Design review of the part built by this model. Coordinates are the model's own, in mm. A direction names the side the tool comes from. Round coordinates to 2 decimals unless told otherwise and drop trailing zeros. Loops run counter-clockwise (first coordinate to the right, second up) from the corner with the lowest first, then second, coordinate; pieces in that order, holes last. Notation, with made-up numbers: (86, -8) -> (128, -8) arc R21 ccw to (128, 29) -> close; hole circle Ø8 at (33, 54). An arc over 180 degrees is marked (long way). Answer as CSV lines item,"result". Start each with the question number.
```python
from build123d import *

# Parameters (mm, degrees)
PAD023_DEPTH     = 30
POCKET022_DEPTH  = 203.460811
POCKET023_DEPTH  = 25.001
SKETCH049_W      = 110.6
SKETCH049_H      = 62.6
POCKET024_DEPTH  = 33.001
SKETCH051_W      = 120.3
SKETCH051_H      = 69.7
POCKET025_DEPTH  = 2
CHAMFER001_SIZE2 = 2
CHAMFER001_SIZE  = 4
SKETCH054_R      = 1.25
POCKET029_DEPTH  = 7.001
SKETCH052_R      = 3
POCKET030_DEPTH  = 3


with BuildPart() as part:
    # Sketch045 → Pad023 (new body)
    with BuildSketch(Plane.XZ.offset(7)):
        with BuildLine():
            ThreePointArc((-100.852547, 31.281341), (-87.977329, 12.342987), (-66.272551, 5.039896))
            Line((-66.272551, 5.039896), (66.272551, 5.039896))
            ThreePointArc((66.272551, 5.039896), (87.977329, 12.342987), (100.852547, 31.281341))
            ThreePointArc((100.852547, 31.281341), (100.091262, 61.855424), (91.843705, 91.305923))
            ThreePointArc((34.688969, 97.850786), (63.036347, 92.569904), (91.843705, 91.305923))
            ThreePointArc((34.688969, 97.850786), (0, 104.060193), (-34.688969, 97.850786))
            ThreePointArc((-91.843705, 91.305923), (-63.036347, 92.569904), (-34.688969, 97.850786))
            ThreePointArc((-91.843705, 91.305923), (-100.091262, 61.855424), (-100.852547, 31.281341))
        make_face()
    extrude(amount=PAD023_DEPTH)

    # Sketch048 → Pocket022 (cut, through all)
    with BuildSketch(Plane.YZ.offset(102)):
        with BuildLine():
            ThreePointArc((-12, 23.34), (-23.12479, 56.152072), (-39.155961, 86.866801))
            Line((-39.155961, 23.34), (-39.155961, 86.866801))
            Line((-39.155961, 23.34), (-12, 23.34))
        make_face()
    extrude(amount=-POCKET022_DEPTH, mode=Mode.SUBTRACT)

    # Sketch050 → Pocket023 (cut, through all)
    with BuildSketch(Plane.XZ.offset(12)):
        with BuildLine():
            ThreePointArc((-86.154363, 83.544791), (-58.846051, 86.250597), (-32.141142, 92.568282))
            ThreePointArc((32.141142, 92.568282), (0, 97.874317), (-32.141142, 92.568282))
            ThreePointArc((32.141142, 92.568282), (58.846051, 86.250597), (86.154363, 83.544791))
            ThreePointArc((93.603594, -14.330003), (97.449111, 35.183555), (86.154363, 83.544791))
            Line((-93.603594, -14.330003), (93.603594, -14.330003))
            ThreePointArc((-86.154363, 83.544791), (-98.508002, 35.264147), (-93.603594, -14.330003))
        make_face()
    extrude(amount=POCKET023_DEPTH, mode=Mode.SUBTRACT)

    # Sketch049 → Pocket024 (cut, through all)
    with BuildSketch(Plane.XZ.offset(4)):
        with Locations((0, 41.080998)):
            Rectangle(SKETCH049_W, SKETCH049_H)
    extrude(amount=POCKET024_DEPTH, mode=Mode.SUBTRACT)

    # Sketch051 → Pocket025 (cut)
    with BuildSketch(Plane(origin=(0, -7, 41), x_dir=(1, 0, 0), z_dir=(0, -1, 0))):
        with Locations((-3.04, -0.08)):
            Rectangle(SKETCH051_W, SKETCH051_H)
    extrude(amount=POCKET025_DEPTH, mode=Mode.SUBTRACT)

    # Chamfer001
    chamfer001_edges = [part.edges().sort_by_distance(p)[0] for p in [
        (55.3, -12, 41.080998),
        (0, -12, 72.380998),
        (-55.3, -12, 41.080998),
        (0, -12, 9.780998),
    ]]
    chamfer001_side = part.faces().sort_by_distance((-83.299387, -12, 11.829323))[0]
    chamfer(chamfer001_edges, length=CHAMFER001_SIZE, length2=CHAMFER001_SIZE2, reference=chamfer001_side)

    # Sketch054 → Pocket029 (cut, through all)
    with BuildSketch(Plane.XZ.offset(14)):
        with Locations((-81.894745, 30.682003)):
            Circle(SKETCH054_R)
        with Locations((-91.343391, 51.252899)):
            Circle(SKETCH054_R)
        with Locations((91.343391, 51.252899)):
            Circle(SKETCH054_R)
        with Locations((81.894745, 30.682003)):
            Circle(SKETCH054_R)
    extrude(amount=-POCKET029_DEPTH, mode=Mode.SUBTRACT)

    # Sketch052 → Pocket030 (cut)
    with BuildSketch(Plane.XZ.offset(12)):
        with Locations((-81.894745, 30.682003)):
            Circle(SKETCH052_R)
        with Locations((81.894745, 30.682003)):
            Circle(SKETCH052_R)
        with Locations((91.343391, 51.252899)):
            Circle(SKETCH052_R)
        with Locations((-91.343391, 51.252899)):
            Circle(SKETCH052_R)
    extrude(amount=-POCKET030_DEPTH, mode=Mode.SUBTRACT)


solid = part.part
```
Q1. Add section B-B, the plane z = 45. Give the boundary of the cut face in (x, y), and give its area (3 significant figures).
Q2. Mouldability with a two-part tool opening along X and no side actions: class faces 1 (the cylindrical face through (-98.807, -18.457, 68.983)), 2 (the flat face through (57.3, -11, 40.6)), 3 (the cylindrical face through (87.72, -9.74, 12.15)) as pulls with the +X half, pulls with the -X half, needs draft (parallel to the pull), parting line crosses it, or undercut.
Q3. Add section A-A, the plane x = -43. Give the boundary of the cut face in (y, z), and give its area (3 significant figures).
Q4. For pin 1 Ø12 at (y, z) = (-18.5, 75) entering from +X; pin 2 Ø5 at (x, z) = (-91.34, 51.25) entering from -Y; pin 3 Ø6 at (y, z) = (-15, 55.5) entering from -X; pin 4 Ø2 at (x, z) = (-91.34, 51.25) entering from +Y, all flat-tipped, find the tip position at first contact; note any pin that passes through.
Q5. Add section C-C, the plane y = -34.5. Give the boundary of the cut face in (x, z), and give its area (3 significant figures).
Q6. To check wall thickness, follow probe 1 along Y at (x, z) = (-23, 88); probe 2 along X at (y, z) = (-30, 73.5); probe 3 along X at (y, z) = (-12.5, 59.5). State the ranges of each line that lie inside material, in increasing order. Write a range as from..to.
Q7. Machinability: for faces 4 (the flat face through (-57, -9, 41)), 5 (the cylindrical face through (-91.734, -10.521, 54.227)), 6 (the cylindrical face through (58.467, -24.325, 86.314)), which of the approach directions +Z, -Z, +X, -X, +Y, -Y give a long, thin tool a straight path to every point of the face, cutting with its end or side? Answer none if there is none.
Q8. Add section D-D, the plane x = -18. Give the boundary of the cut face in (y, z), and give its area (3 significant figures).
Worked answers:
1,outline,"(-101.45, -18.71) -> (-97.43, -18.71) -> (-97.43, -12) -> (-59.3, -12) -> (-55.3, -10) -> (-55.3, -9) -> (-63.19, -9) -> (-63.19, -7) -> (-101.45, -7) -> close; (55.3, -10) -> (59.3, -12) -> (96.4, -12) -> (96.4, -18.71) -> (101.45, -18.71) -> (101.45, -7) -> (57.11, -7) -> (57.11, -9) -> (55.3, -9) -> close"
1,area,"495 mm^2"
2,face 1,"pulls with the -X half"
2,face 2,"undercut"
2,face 3,"pulls with the +X half"
3,outline,"(-37, 89.54) -> (-12, 89.54) -> (-12, 76.38) -> (-10, 72.38) -> (-9, 72.38) -> (-9, 75.77) -> (-7, 75.77) -> (-7, 95.87) -> (-37, 95.87) -> close; (-12, 5.04) -> (-7, 5.04) -> (-7, 6.07) -> (-9, 6.07) -> (-9, 9.78) -> (-10, 9.78) -> (-12, 5.78) -> close"
3,area,"277 mm^2"
4,pin 1,"stops at x = 98.8"
4,pin 2,"stops at y = -9"
4,pin 3,"stops at x = -101.13"
4,pin 4,"passes through"
5,outline,"(-96.24, 79.06) -> (-88.09, 79.06) arc R143.5 cw to (-86.15, 83.54) arc R205.65 ccw to (-32.14, 92.57) arc R100 cw to (32.14, 92.57) arc R205.65 ccw to (86.15, 83.54) arc R162.43 cw to (87.88, 79.06) -> (96.24, 79.06) arc R123.56 ccw to (91.84, 91.31) arc R205.65 cw to (34.69, 97.85) arc R100 ccw to (-34.69, 97.85) arc R205.65 cw to (-91.84, 91.31) arc R123.56 ccw to start"
5,area,"1,320 mm^2"
6,probe 1,"y = -12..-7"
6,probe 2,"x = -97.77..-90.25, 89.82..97.77"
6,probe 3,"x = -100.42..-94.56, 93.73..100.42"
7,face 4,"+Y"
7,face 5,"-Y"
7,face 6,"-Z, -Y"
8,outline,"(-37, 96.24) -> (-12, 96.24) -> (-12, 76.38) -> (-10, 72.38) -> (-9, 72.38) -> (-9, 75.77) -> (-7, 75.77) -> (-7, 102.43) -> (-37, 102.43) -> close; (-12, 5.04) -> (-7, 5.04) -> (-7, 6.07) -> (-9, 6.07) -> (-9, 9.78) -> (-10, 9.78) -> (-12, 5.78) -> close"
8,area,"306 mm^2"
